from build123d import *

# Parameters (mm, degrees)
SKETCH1_R = 7.5


with BuildPart() as part:
    # Sweep3: sweep along a curve in space
    with BuildLine() as sweep3_path:
        Line((0, 0, 0), (-112.552079249, 0, 0))
        ThreePointArc((-112.552079249, 0, 0), (-116.378913573, 0.761204675, 0), (-119.623147061, 2.928932188, 0))
        Line((-119.623147061, 2.928932188, 0), (-184.039505872, 67.345290999, 0))
        ThreePointArc((-184.039505872, 67.345290999, 0), (-187.28373936, 69.513018512, 0), (-191.110573684, 70.274223187, 0))
        Line((-191.110573684, 70.274223187, 0), (-285.776779589, 70.274223187, 0))
        ThreePointArc((-285.776779589, 70.274223187, 0), (-292.977279683, 67.213444929, 0), (-295.769952951, 59.904782865, 0))
        Line((-295.769952951, 59.904782865, 0), (-292.90806011, -17.507967024, 0))
    # Sketch1 → Sweep3 (sweep)
    with BuildSketch(Plane(origin=(0, 0, 0), x_dir=(0, 0, -1), z_dir=(1, 0, 0))):
        Circle(SKETCH1_R)
    sweep(path=sweep3_path.line)


solid = part.part
Verification items for the finished model (mm, model axes). A direction names the side the tool comes from. Coordinates: 2 decimals unless noted, no trailing zeros. Write each loop counter-clockwise with the first axis right and the second up, starting at its lowest first coordinate (ties: lowest second). Pieces come first, ordered by that corner, then holes. Notation, with made-up numbers: (-8.75, 65) - (46.25, 65) arc R14 ccw to (46.25, 70) - close; hole circle Ø5 at (1, 4.25). An arc over 180 degrees is marked (long way). Answer as a JSON object with one key per item and string values.
(1) Tool access check on faces 5 (the cylindrical face through (-57.064, -0.33, 7.493)), 6 (the cylindrical face through (-239.1, 77.6, 1.6)). Record the directions out of +Z, -Z, +X, -X, +Y, -Y that give a thin tool (end or side, any length) a straight path to the whole face; none if there is none.
Report:
{"face 5": "+X", "face 6": "none"}
(2) Gauge pin test, flat ends, axial feed: pin 1 Ø5 at (y, z) = (24.5, -5.5) entering from -X; pin 2 Ø2 at (y, z) = (20.5, 0) entering from -X; pin 3 Ø1 at (x, y) = (-120, -4.5) entering from +Z; pin 4 Ø8 at (x, y) = (-196, 67.5) entering from -Z. Record the tip position at first contact, or that the pin passes through.
Report:
{"pin 1": "x = -301.34", "pin 2": "x = -301.86", "pin 3": "z = 4.75", "pin 4": "z = -7.5"}
(3) Mould release check, pull along Y, two halves, no side actions. Record for faces 1 (the flat face through (0, 0, 0)), 2 (the cylindrical face through (-301.636, 20.386, 1.626)), 3 (the cylindrical face through (-147.11, 40.77, 1.63)), 4 (the flat face through (-293.01, -17.51, -0.11)): pulls with the +Y half, pulls with the -Y half, needs draft (parallel to the pull), parting line crosses it, or undercut.
Report:
{"face 1": "needs draft", "face 2": "undercut", "face 3": "parting line crosses it", "face 4": "pulls with the -Y half"}
(4) Cross-section at B-B on x = -250. Record the cut outline in (y, z).
Report:
{"outline": "circle Ø15 at (70.27, 0)"}
(5) Thickness scan on line 1 along X through (y, z) = (37, 4.75); line 2 along X through (y, z) = (28, -4.5); line 3 along Z through (x, y) = (-36.5, -1). Record the ranges inside material, lowest first.
Report:
{"line 1": "-300.73 to -289.12, -161.9 to -145.49", "line 2": "-300.59 to -288.59, -153.18 to -136.21", "line 3": "-7.43 to 7.43"}
(6) Cross-section at A-A on z = -3. Record the cut outline in (x, y).
Report:
{"outline": "(-302.64, 59.65) - (-299.78, -17.76) - (-286.04, -17.25) - (-288.9, 60.16) arc R3.13 cw to (-285.78, 63.4) - (-191.11, 63.4) arc R3.13 cw to (-188.9, 62.48) - (-124.48, -1.93) arc R16.87 ccw to (-112.55, -6.87) - (0, -6.87) - (0, 6.87) - (-112.55, 6.87) arc R3.13 cw to (-114.76, 7.79) - (-179.18, 72.21) arc R16.87 ccw to (-191.11, 77.15) - (-285.78, 77.15) arc R16.87 ccw to start"}
